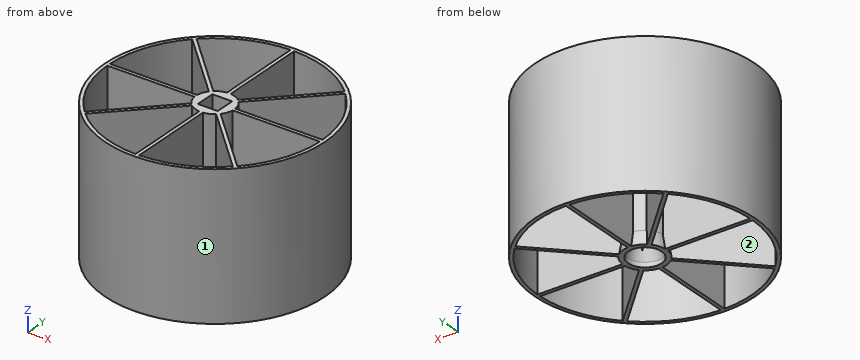
from build123d import *

# Parameters (mm, degrees)
CYLINDER014_R          = 7
CYLINDER014_DEPTH      = 2
TUBE015_R              = 60
TUBE015_R_2            = 46
TUBE015_DEPTH          = 60
BOX004_W               = 8.3
BOX004_H               = 8.3
BOX004_DEPTH           = 60
BOX003_W               = 100
BOX003_H               = 1.5
BOX003_DEPTH           = 60
CYLINDER001_R          = 8
CYLINDER001_DEPTH      = 60
TUBE_R                 = 46
TUBE_R_2               = 44.5
TUBE_DEPTH             = 60
BOX024_W               = 100
BOX024_H               = 1.5
BOX024_DEPTH           = 60
BOX024_PLACEMENT_ANGLE = 45
BOX025_W               = 100
BOX025_H               = 1.5
BOX025_DEPTH           = 60
BOX025_PLACEMENT_ANGLE = 135
BOX_W                  = 100
BOX_H                  = 1.5
BOX_DEPTH              = 60


with BuildPart() as cone:
    # Cone → Cone (revolve)
    with BuildSketch(Plane(origin=(0, 0, 2), x_dir=(1, 0, 0), z_dir=(0, -1, 0))):
        Polygon((0, 0), (7, 0), (4, 10), (0, 10), align=None)
    revolve(axis=Axis((0, 0, 2), (0, 0, 1)))


with BuildPart() as cylinder014:
    # Cylinder014 → Cylinder014 (new body)
    with BuildSketch(Plane.XY):
        Circle(CYLINDER014_R)
    extrude(amount=CYLINDER014_DEPTH)


with BuildPart() as tube015:
    # Tube015 → Tube015 (new body)
    with BuildSketch(Plane.XY):
        Circle(TUBE015_R)
        Circle(TUBE015_R_2, mode=Mode.SUBTRACT)
    extrude(amount=TUBE015_DEPTH)


with BuildPart() as fusion001:
    # Box004 → Box004 (new body)
    with BuildSketch(Plane(origin=(-4.15, -4.15, 0), x_dir=(1, 0, 0), z_dir=(0, 0, 1))):
        with Locations((4.15, 4.15)):
            Rectangle(BOX004_W, BOX004_H)
    extrude(amount=BOX004_DEPTH)

    # Fusion001: union Cone, Cylinder014, Tube015
    add(cone.part)
    add(cylinder014.part)
    add(tube015.part)


with BuildPart() as cube003:
    # Box003 → Box003 (new body)
    with BuildSketch(Plane(origin=(-0.8, 48.5, 0), x_dir=(0, -1, 0), z_dir=(0, 0, 1))):
        with Locations((50, 0.75)):
            Rectangle(BOX003_W, BOX003_H)
    extrude(amount=BOX003_DEPTH)


with BuildPart() as cylinder001:
    # Cylinder001 → Cylinder001 (new body)
    with BuildSketch(Plane.XY):
        Circle(CYLINDER001_R)
    extrude(amount=CYLINDER001_DEPTH)


with BuildPart() as tube:
    # Tube → Tube (new body)
    with BuildSketch(Plane.XY):
        Circle(TUBE_R)
        Circle(TUBE_R_2, mode=Mode.SUBTRACT)
    extrude(amount=TUBE_DEPTH)


with BuildPart() as cone001:
    # Cone001 → Cone001 (revolve)
    with BuildSketch(Plane.XZ):
        Polygon((0, 0), (9, 0), (4, 30), (0, 30), align=None)
    revolve(axis=Axis((0, 0, 0), (0, 0, 1)))


with BuildPart() as cube024:
    # Box024 → Box024 (new body)
    with BuildSketch(Plane.XY):
        with Locations((50, 0.75)):
            Rectangle(BOX024_W, BOX024_H)
    extrude(amount=BOX024_DEPTH)


with BuildPart() as cube024_1:
    # Box024 placement: moved
    add(cube024.part.moved(Location((-32.999286, -34.092597, 0))).rotate(Axis((-32.999286, -34.092597, 0), (0, 0, 1)), BOX024_PLACEMENT_ANGLE))


with BuildPart() as cube025:
    # Box025 → Box025 (new body)
    with BuildSketch(Plane.XY):
        with Locations((50, 0.75)):
            Rectangle(BOX025_W, BOX025_H)
    extrude(amount=BOX025_DEPTH)


with BuildPart() as cube025_1:
    # Box025 placement: moved
    add(cube025.part.moved(Location((34.387991, -33.456201, 0))).rotate(Axis((34.387991, -33.456201, 0), (0, 0, 1)), BOX025_PLACEMENT_ANGLE))


with BuildPart() as obj1:
    # Box → Box (new body)
    with BuildSketch(Plane(origin=(-47, -0.8, 0), x_dir=(1, 0, 0), z_dir=(0, 0, 1))):
        with Locations((50, 0.75)):
            Rectangle(BOX_W, BOX_H)
    extrude(amount=BOX_DEPTH)

    # Fusion: union Cube003, Cylinder001, Tube, Cone001, Cube024, Cube025
    add(cube003.part)
    add(cylinder001.part)
    add(tube.part)
    add(cone001.part)
    add(cube024_1.part)
    add(cube025_1.part)

    # Cut: cut Fusion001
    add(fusion001.part, mode=Mode.SUBTRACT)


with BuildPart() as obj1_1:
    # Cut placement: moved
    add(obj1.part.moved(Location((0, 0, 2.5))))


solid = obj1_1.part
Can you work these out from the model? Positions are in its coordinate system, mm. Face numbers are marked on the shaded views. Round coordinates to 2 decimals unless told otherwise and drop trailing zeros. Write each loop counter-clockwise with the first axis right and the second up, starting at its lowest first coordinate (ties: lowest second). Pieces come first, ordered by that corner, then holes. Notation, with made-up numbers: (50.5, 44.5) -> (78.5, 44.5) arc R14 cw to (78.5, 65.5) -> close; hole circle Ø7 at (70.5, 49). An arc over 180 degrees is marked (long way). Use one line per item in the form item = value. Start each with the question number.
Q1. Imagine slicing it at B-B (x = -24.5). Please give me the cut outline in (y, z).
Q2. Imagine slicing it at A-A (y = -27). Please give me the cut outline in (x, z).
Q3. If I drill on probe 1 along Y at (x, z) = (0, 3.4); probe 2 along X at (y, z) = (-29, 36); probe 3 along X at (y, z) = (23, 28.5), over which ranges is the centre line in solid material (lowest first)? Write a range as [from, to].
Q4. I'm going to push flat-ended pins straight in: P1, Ø10, axis at x = 1.5, z = 36.5, coming from the -Y side; P2, Ø18.5, axis at y = 28.5, z = 38, coming from the -X side; P3, Ø2, axis at x = 27, z = 26, coming from the -Y side. Where does each tip first touch, or does it pass through?
Q5. Imagine slicing it at C-C (z = 49.5). Count the separate pieces of the cut face and the enclosed holes in it, then the cut area to 3 significant figures.
Q6. We'd pull the mould along Y, two halves only. Please class the marked faces 1 and 2: +Y half, -Y half, draft (parallel to the pull), parting line (faces both ways), or undercut.
Worked out:
q1.outline = (-38.93, 2.5) -> (-37.15, 2.5) -> (-37.15, 62.5) -> (-38.93, 62.5) -> close; (-25.59, 2.5) -> (-23.47, 2.5) -> (-23.47, 62.5) -> (-25.59, 62.5) -> close; (-0.8, 2.5) -> (0.7, 2.5) -> (0.7, 62.5) -> (-0.8, 62.5) -> close; (23.31, 2.5) -> (25.43, 2.5) -> (25.43, 62.5) -> (23.31, 62.5) -> close; (37.15, 2.5) -> (38.93, 2.5) -> (38.93, 62.5) -> (37.15, 62.5) -> close
q2.outline = (-37.24, 2.5) -> (-35.37, 2.5) -> (-35.37, 62.5) -> (-37.24, 62.5) -> close; (-28.03, 2.5) -> (-25.91, 2.5) -> (-25.91, 62.5) -> (-28.03, 62.5) -> close; (-0.8, 2.5) -> (0.7, 2.5) -> (0.7, 62.5) -> (-0.8, 62.5) -> close; (25.81, 2.5) -> (27.93, 2.5) -> (27.93, 62.5) -> (25.81, 62.5) -> close; (35.37, 2.5) -> (37.24, 2.5) -> (37.24, 62.5) -> (35.37, 62.5) -> close
q3.probe_1 = [-46, -7], [7, 46]
q3.probe_2 = [-35.71, -33.75], [-30.03, -27.91], [-0.8, 0.7], [27.81, 29.93], [33.75, 35.71]
q3.probe_3 = [-39.84, -38.1], [-24.19, -22.07], [-0.8, 0.7], [21.97, 24.09], [38.1, 39.84]
q4.P1 = -46
q4.P2 = -41.78
q4.P3 = -37.95
q5.separate_pieces = 1
q5.enclosed_holes = 9
q5.area = 997 mm^2
q6.face_1 = parting line
q6.face_2 = undercut
